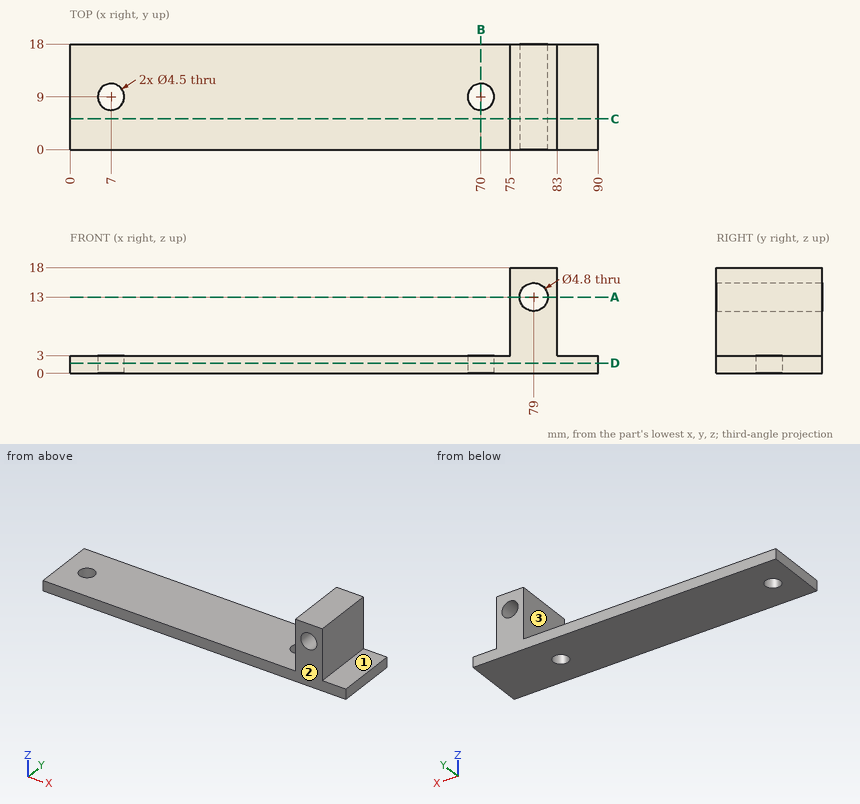
Verification items for this drawing (mm, ordinates from the low corner). A direction names the side the tool comes from. Coordinates: 2 decimals unless noted, no trailing zeros. Loops run counter-clockwise (first coordinate to the right, second up) from the corner with the lowest first, then second, coordinate; pieces in that order, holes last. Notation, with made-up numbers: (17.5, 60.25) - (50.5, 60.25) arc R16 ccw to (50.5, 79.25) - close; hole circle Ø10 at (-6.75, -13). An arc over 180 degrees is marked (long way). Answer as a JSON object with one key per item and string values.
(1) Go/stop test with flat-tipped pins: pin 1 Ø2 at (x, y) = (88, 13) entering from +Z; pin 2 Ø1 at (x, z) = (74, 6) entering from +Y; pin 3 Ø3 at (x, z) = (77.5, 2.5) entering from -Y; pin 4 Ø4 at (y, z) = (5.5, 8.5) entering from +X. Record where each tip stops, or that it passes through.
Response:
{"pin 1": "stops at z = 3", "pin 2": "passes through", "pin 3": "stops at y = 0", "pin 4": "stops at x = 83"}
(2) Cross-section at B-B, the plane x = 70. Record the boundary of the cut face in (y, z), then the cut area to 3 significant figures.
Response:
{"outline": "(0, 0) - (6.75, 0) - (6.75, 3) - (0, 3) - close; (11.25, 0) - (18, 0) - (18, 3) - (11.25, 3) - close", "area": "40.5 mm²"}
(3) Scan lines: line 1 along Y through (x, z) = (7, 0.95); line 2 along Z through (x, y) = (43.5, 12.25); line 3 along X through (y, z) = (1.5, 17.25). Record each from-to range of solid material in increasing order.
Response:
{"line 1": "y = 0 to 6.75, 11.25 to 18", "line 2": "z = 0 to 3", "line 3": "x = 75 to 83"}
(4) Access from +Z, -Z, +X, -X, +Y, -Y to the whole of each face (thin tool, end or side, straight path). Record for the marked faces 1, 2 and 3.
Response:
{"face 1": "+Z, +X, +Y, -Y", "face 2": "+Z, -Z, +X, -X, -Y", "face 3": "+Z, -X, +Y, -Y"}
(5) Cross-section at D-D, the plane z = 1.75. Record the boundary of the cut face in (x, y), then the cut area to 3 significant figures.
Response:
{"outline": "(0, 0) - (90, 0) - (90, 18) - (0, 18) - close; hole circle Ø4.5 at (7, 9); hole circle Ø4.5 at (70, 9)", "area": "1,590 mm²"}
(6) Cross-section at A-A, the plane z = 13. Record the boundary of the cut face in (x, y), then the cut area to 3 significant figures.
Response:
{"outline": "(75, 0) - (76.6, 0) - (76.6, 18) - (75, 18) - close; (81.4, 0) - (83, 0) - (83, 18) - (81.4, 18) - close", "area": "57.6 mm²"}
(7) Cross-section at C-C, the plane y = 5.25. Record the boundary of the cut face in (x, z), then the cut area to 3 significant figures.
Response:
{"outline": "(0, 0) - (90, 0) - (90, 3) - (83, 3) - (83, 18) - (75, 18) - (75, 3) - (0, 3) - close; hole circle Ø4.8 at (79, 13)", "area": "372 mm²"}
